Source: CAD feature listing. Evaluate the final solid. Frame: model axes, mm. A direction names the side the tool comes from. Coordinates: 2 decimals unless noted, no trailing zeros. Loops run counter-clockwise (first coordinate to the right, second up) from the corner with the lowest first, then second, coordinate; pieces in that order, holes last. Notation, with made-up numbers: M 30.25,82 L 44.25,82 A25 cw 44.25,103 Z; hole C 59.25,60.25 d10. An arc over 180 degrees is marked long. One line per question, with ' | ' between items. Start each with the question number.
1. Access query for faces 1 (the flat face through (10, 0, 30)), 2 (the flat face through (0, 11, 33)), 3 (the flat face through (6.25, 14, 18)), 4 (the flat face through (-10, 11, 18)), 5 (the cylindrical face through (-0.4, 8.4, 2.5)). Directions: +Z, -Z, +X, -X, +Y, -Y. A direction counts if a zero-diameter tool reaches every point of the face in a straight line with its end or side. Return the directions, or none.
2. Section query B-B, the plane y = 0. Output: boundary loops of the cut face in (x, z).
3. Section query C-C, the plane x = -5.5. Output: boundary loops of the cut face in (y, z), and give its area (3 significant figures).
4. Ray query, probe 1 along Y at (x, z) = (0, 4); probe 2 along X at (y, z) = (10, 2.35); probe 3 along X at (y, z) = (-7.5, 31). Return the intervals inside material, ascending.
5. Mould query, pull axis X, two halves, no side actions, for faces 6 (the flat face through (14.25, 0, 34)), 7 (the flat face through (-10, -11, 18)), 8 (the flat face through (-4, 0, 5)). Classes: pulls with the +X half, pulls with the -X half, needs draft (parallel to the pull), parting line crosses it, or undercut.
6. Section query A-A, the plane z = 26.5. Output: boundary loops of the cut face in (x, y), and give its area (3 significant figures).
7. Pin query (flat end, axial travel): P1, Ø4, axis at x = -1, y = -14, coming from the +Z side; P2, Ø10, axis at y = -1, z = 7, coming from the +X side. Return the tip coordinate at first contact, or that it passes through.
8. Section query D-D, the plane x = 0. Output: boundary loops of the cut face in (y, z).
```python
from build123d import *

# Parameters (mm, degrees)
SKETCH_1_W          = 28.5
SKETCH_1_H          = 32
EXTRUDE_1_DEPTH     = 5
SKETCH_3_R          = 2
EXTRUDE_2_DEPTH     = 8
SKETCH_4_R          = 1.65
CUT_EXTRUDE_1_DEPTH = 6
SKETCH_5_R          = 1.65
CUT_EXTRUDE_2_DEPTH = 5
SKETCH_6_W          = 25
SKETCH_6_H          = 22
CUT_EXTRUDE_3_DEPTH = 29.5
EXTRUDE_3_REACH     = 22.5
SKETCH_7_W          = 5
SKETCH_7_H          = 5
SKETCH_8_W          = 8
SKETCH_8_H          = 22
CUT_EXTRUDE_4_DEPTH = 10


with BuildPart() as part:
    # ｽｹｯﾁ1 → ﾎﾞｽ - 押し出し1 (new body)
    with BuildSketch(Plane.XY):
        Rectangle(SKETCH_1_W, SKETCH_1_H)
    extrude(amount=EXTRUDE_1_DEPTH)

    # ｽｹｯﾁ3 → ﾎﾞｽ - 押し出し2 (add)
    with BuildSketch(Plane(origin=(14.25, 0, 0), x_dir=(0, 0, -1), z_dir=(1, 0, 0))):
        with BuildLine():
            Line((-5, 16), (-35, 16))
            Line((-35, 16), (-52.772001082, 4.161251014))
            ThreePointArc((-52.772001082, 4.161251014), (-55, 0), (-52.772001082, -4.161251014))
            Line((-52.772001082, -4.161251014), (-35, -16))
            Line((-35, -16), (-5, -16))
            Line((-5, -16), (-5, 16))
        make_face()
        with Locations((-50, 0)):
            Circle(SKETCH_3_R, mode=Mode.SUBTRACT)
    extrude_2 = extrude(amount=-EXTRUDE_2_DEPTH)

    # ﾐﾗｰ1: ﾎﾞｽ - 押し出し2 across plane
    add(extrude_2.mirror(Plane(origin=(0, 0, 0), x_dir=(0, 0, 1), z_dir=(1, 0, 0))))

    # ｽｹｯﾁ4 → ｶｯﾄ - 押し出し1 (cut, through all)
    with BuildSketch(Plane.XY.offset(5)):
        with Locations((0, 10)):
            Circle(SKETCH_4_R)
        with Locations((0, -10)):
            Circle(SKETCH_4_R)
    extrude(amount=-CUT_EXTRUDE_1_DEPTH, mode=Mode.SUBTRACT)

    # ｽｹｯﾁ5 → ｶｯﾄ - 押し出し2 (cut)
    with BuildSketch(Plane.XY):
        with Locations((12.35, -5)):
            Circle(SKETCH_5_R)
        with Locations((12.35, 5)):
            Circle(SKETCH_5_R)
    extrude(amount=CUT_EXTRUDE_2_DEPTH, mode=Mode.SUBTRACT)

    # ｽｹｯﾁ6 → ｶｯﾄ - 押し出し3 (cut, through all)
    with BuildSketch(Plane(origin=(14.25, 0, 0), x_dir=(0, 0, -1), z_dir=(1, 0, 0))):
        with Locations((-17.5, 0)):
            Rectangle(SKETCH_6_W, SKETCH_6_H)
    extrude(amount=-CUT_EXTRUDE_3_DEPTH, mode=Mode.SUBTRACT)

    # ｽｹｯﾁ7 → ﾎﾞｽ - 押し出し3 (add, up to next)
    with BuildSketch(Plane(origin=(-6.25, 0, 0), x_dir=(0, 0, -1), z_dir=(1, 0, 0)), mode=Mode.PRIVATE) as extrude_3_sk1:
        with Locations((-32.5, 13.5)):
            Rectangle(SKETCH_7_W, SKETCH_7_H)
    extrude_3_tool1 = extrude(extrude_3_sk1.sketch, amount=EXTRUDE_3_REACH, mode=Mode.PRIVATE) - part.part
    add(extrude_3_tool1.solids().sort_by_distance((-6.25, 13.5, 32.5))[0])
    # ｽｹｯﾁ7 → ﾎﾞｽ - 押し出し3 (add, up to next)
    with BuildSketch(Plane(origin=(-6.25, 0, 0), x_dir=(0, 0, -1), z_dir=(1, 0, 0)), mode=Mode.PRIVATE) as extrude_3_sk2:
        with Locations((-32.5, -13.5)):
            Rectangle(SKETCH_7_W, SKETCH_7_H)
    extrude_3_tool2 = extrude(extrude_3_sk2.sketch, amount=EXTRUDE_3_REACH, mode=Mode.PRIVATE) - part.part
    add(extrude_3_tool2.solids().sort_by_distance((-6.25, -13.5, 32.5))[0])

    # ｽｹｯﾁ8 → ｶｯﾄ - 押し出し4 (cut)
    with BuildSketch(Plane(origin=(0, 0, 0), x_dir=(-1, 0, 0), z_dir=(0, 0, -1))):
        with Locations((-10.25, 0)):
            Rectangle(SKETCH_8_W, SKETCH_8_H)
    extrude(amount=-CUT_EXTRUDE_4_DEPTH, mode=Mode.SUBTRACT)


solid = part.part
```
Taken from the geometry:
1) face 1: -Z, +X, -X | face 2: +Z | face 3: +Y, -Y | face 4: +X, -X | face 5: -Z
2) outline: M -14.25,0 L 6.25,0 L 6.25,5 L -14.25,5 Z; M -14.25,30 L -6.25,30 L -6.25,48 L -14.25,48 Z; M -14.25,52 L -6.25,52 L -6.25,55 L -14.25,55 Z; M 6.25,30 L 14.25,30 L 14.25,48 L 6.25,48 Z; M 6.25,52 L 14.25,52 L 14.25,55 L 6.25,55 Z
3) outline: M -16,0 L 16,0 L 16,5 L -16,5 Z; M -16,30 L -11,30 L -11,35 L -16,35 Z; M 11,30 L 16,30 L 16,35 L 11,35 Z | area: 210 mm^2
4) probe 1: -16 to -11.65, -8.35 to 8.35, 11.65 to 16 | probe 2: -14.25 to -1.65, 1.65 to 6.25 | probe 3: -14.25 to -6.25, 6.25 to 14.25
5) face 6: pulls with the +X half | face 7: needs draft | face 8: undercut
6) outline: M -14.25,-16 L -6.25,-16 L -6.25,-11 L -14.25,-11 Z; M -14.25,11 L -6.25,11 L -6.25,16 L -14.25,16 Z; M 6.25,-16 L 14.25,-16 L 14.25,-11 L 6.25,-11 Z; M 6.25,11 L 14.25,11 L 14.25,16 L 6.25,16 Z | area: 160 mm^2
7) P1: z = 35 | P2: x = 6.25
8) outline: M -16,0 L -11.65,0 L -11.65,5 L -16,5 Z; M -16,30 L -11,30 L -11,35 L -16,35 Z; M -8.35,0 L 8.35,0 L 8.35,5 L -8.35,5 Z; M 11,30 L 16,30 L 16,35 L 11,35 Z; M 11.65,0 L 16,0 L 16,5 L 11.65,5 Z
